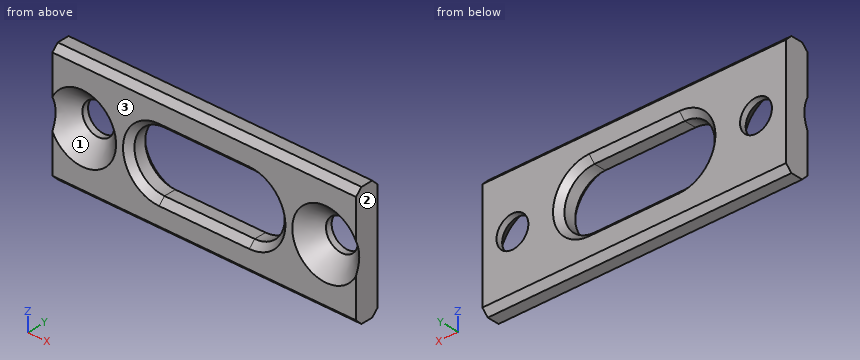
```python
from build123d import *

# Parameters (mm, degrees)
F0_W           = 50.5
F0_H           = 20
F1_DEPTH       = 4
F3_D           = 5.3
F3_DEPTH       = 8
F3_CSINK_D     = 11.2
F3_CSINK_ANGLE = 90
F3_TIP         = 1.5922806404
F5_DEPTH       = 4.001
F6_SIZE        = 1


with BuildPart() as f1:
    # F0 (on Front) → F1 (new body)
    with BuildSketch(Plane.XZ):
        with Locations((0, -10)):
            Rectangle(F0_W, F0_H)
    extrude(amount=F1_DEPTH)

    # F3
    with Locations(Plane.XZ.offset(4)):
        with Locations((-20.25, -10), (20.25, -10)):
            CounterSinkHole(F3_D / 2, F3_CSINK_D / 2, depth=F3_DEPTH, counter_sink_angle=F3_CSINK_ANGLE)
            with Locations((0, 0, -(F3_DEPTH + F3_TIP / 2))):  # 118° drill point
                Cone(0, F3_D / 2, F3_TIP, mode=Mode.SUBTRACT)

    # F4 (on face) → F5 (cut, through all)
    with BuildSketch(Plane.XZ.offset(4)):
        with BuildLine():
            Line((7.5, -5), (-7.5, -5))
            ThreePointArc((-7.5, -5), (-12.5, -10), (-7.5, -15))
            Line((-7.5, -15), (7.5, -15))
            ThreePointArc((7.5, -15), (12.5, -10), (7.5, -5))
        make_face()
    extrude(amount=-F5_DEPTH, mode=Mode.SUBTRACT)

    # F6
    f6_edges = [f1.edges().sort_by_distance(p)[0] for p in [
        (0, -4, -20),
        (0, -4, 0),
        (0, -4, -15),
        (0, 0, -15),
        (0, 0, -20),
        (0, 0, 0),
    ]]
    chamfer(f6_edges, length=F6_SIZE)


solid = f1.part
```
Source: CAD feature listing. Evaluate the final solid. Frame: model axes, mm. Face numbers are marked on the shaded views. Round coordinates to 2 decimals unless told otherwise and drop trailing zeros. Loops run counter-clockwise (first coordinate to the right, second up) from the corner with the lowest first, then second, coordinate; pieces in that order, holes last.
1. Contact query for a flat-ended pin moving along its axis: pin 1 (4 mm diameter, centred on x = -19.5, z = -11, fed in from -Y). Output: stop coordinate, or through.
2. Ray query, L1, parallel to Z at x = 0, y = -2.55; L2, parallel to X at y = -0.45, z = -10; L3, parallel to X at y = -0.35, z = -11. Return the intervals inside material, ascending.
3. Section query C-C on x = -20.25. Output: boundary loops of the cut face in (y, z), and give its area (3 significant figures).
4. Section query A-A on x = -1.5. Output: boundary loops of the cut face in (y, z), and give its area (3 significant figures).
5. Section query B-B on y = -2.45. Output: boundary loops of the cut face in (x, z), and give its area (3 significant figures).
6. Mould query, pull axis X, two halves, no side actions, for the marked faces 1, 2 and 3. Classes: released by +X, released by -X, zero draft, split by the parting line, or undercut.
Answers below:
1. pin 1: stops at y = -1.65
2. L1: z = -20 to -15, -5 to 0
2. L2: x = -25.25 to -22.9, -17.6 to -13.05, 13.05 to 17.6, 22.9 to 25.25
2. L3: x = -25.25 to -22.7, -17.8 to -13.06, 13.06 to 17.8, 22.7 to 25.25
3. outline: (-4, -19) - (-3, -20) - (-1, -20) - (0, -19) - (0, -12.65) - (-1.05, -12.65) - (-4, -15.6) - close; (-4, -4.4) - (-1.05, -7.35) - (0, -7.35) - (0, -1) - (-1, 0) - (-3, 0) - (-4, -1) - close
3. area: 48.1 mm2
4. outline: (-4, -19) - (-3, -20) - (-1, -20) - (0, -19) - (0, -16) - (-1, -15) - (-3, -15) - (-4, -16) - close; (-4, -4) - (-3, -5) - (-1, -5) - (0, -4) - (0, -1) - (-1, 0) - (-3, 0) - (-4, -1) - close
4. area: 36.0 mm2
5. outline: (-25.25, -20) - (25.25, -20) - (25.25, 0) - (-25.25, 0) - close; hole circle Ø8.1 at (-20.25, -10); hole (-7.5, -15) - (7.5, -15) arc R5 ccw to (7.5, -5) - (-7.5, -5) arc R5 ccw to start; hole circle Ø8.1 at (20.25, -10)
5. area: 678 mm2
6. face 1: undercut
6. face 2: released by +X
6. face 3: zero draft
